Here's how the part is built. I have some questions about the finished solid (model axes, mm). A direction names the side the tool comes from. Round coordinates to 2 decimals unless told otherwise and drop trailing zeros. Order: outer loops, then holes, each group sorted by start corner. A loop starts at its lowest first (then second) coordinate and runs counter-clockwise, first axis right, second up. Notation, with made-up numbers: (-5.75, 13.25) - (22.25, 13.25) arc R10 cw to (22.25, 30.25) - close; hole circle Ø6 at (38, 62.5). An arc over 180 degrees is marked (long way). Answer as a JSON object with one key per item and string values.
```python
from build123d import *

# Parameters (mm, degrees)
F0_R         = 74.0650481318
F0_R_2       = 64.8450067866
F1_DEPTH     = 12.7
F2_DEPTH     = 7.62
F0_R_3       = 8.5707717009
F3_DEPTH     = 10.922
F4_R         = 5.08
F5_T4_DEPTH  = 123.6076762244
F5_T11_DEPTH = 122.6061545132
F5_T18_DEPTH = 115.6407516409


# Not quite as in the source:
# - a fillet or chamfer that OpenCascade refuses, or shapes differently, is made with other operations: its cross-section is extruded or revolved along the edge and cut away or added


with BuildPart() as f1:
    # F0 (on Top) → F1 (new body)
    with BuildSketch(Plane.XY):
        Circle(F0_R)
        Circle(F0_R_2, mode=Mode.SUBTRACT)
    extrude(amount=F1_DEPTH)

    # F0 (on Top) → F2 (join)
    with BuildSketch(Plane.XY):
        Circle(F0_R_2)
        Polygon((45.8412840962, -32.8662097454), (-43.6711683869, -32.8662097454), (0, 53.1617254019), align=None, mode=Mode.SUBTRACT)
    extrude(amount=F2_DEPTH)

    # F0 (on Top) → F3 (join)
    with BuildSketch(Plane.XY):
        Polygon((0, 53.1617254019), (-43.6711683869, -32.8662097454), (45.8412840962, -32.8662097454), align=None)
        Circle(F0_R_3, mode=Mode.SUBTRACT)
    extrude(amount=F3_DEPTH)

    # F4
    f4_edges = [f1.edges().sort_by_distance(p)[0] for p in [
        (-74.065048, 0, 12.7),
    ]]
    fillet(f4_edges, radius=F4_R)

    # F5: chamfer of 5.08 on 4 edges, made by hand


with BuildPart() as f5_tool2:
    # F5_s3 → F5_t4 (new body)
    with BuildSketch(Plane(origin=(29.9216472697, -56.1523871237, 0), x_dir=(0, 0, 1), z_dir=(-0.4702664859, 0.8825244655, 0))):
        Polygon((10.922, 19.9201777866), (5.842, 25.0001777866), (10.922, 25.0001777866), align=None)
    extrude(amount=F5_T4_DEPTH)

    split(bisect_by=Plane.XY.offset(7.62), keep=Keep.TOP)

    split(bisect_by=Plane(origin=(-21.4574493748, 10.8926464781, 0), x_dir=(0, 0, 1), z_dir=(0.8916858157, -0.4526548422, 0)), keep=Keep.TOP)

    split(bisect_by=Plane.XZ.offset(32.8662097454), keep=Keep.BOTTOM)


with BuildPart() as f1_1:
    add(f1.part)

    # F5_t1: cut F5_tool2
    add(f5_tool2.part, mode=Mode.SUBTRACT)


with BuildPart() as f5_tool9:
    # F5_s10 → F5_t11 (new body)
    with BuildSketch(Plane(origin=(27.3709999402, 53.9181957971, 0), x_dir=(0, 0, 1), z_dir=(-0.4526548422, -0.8916858157, 0))):
        Polygon((10.922, 18.9839124202), (5.842, 24.0639124202), (10.922, 24.0639124202), align=None)
    extrude(amount=F5_T11_DEPTH)

    split(bisect_by=Plane.XY.offset(7.62), keep=Keep.TOP)

    split(bisect_by=Plane(origin=(22.0632685396, 11.7567457534, 0), x_dir=(0, 0, 1), z_dir=(-0.8825244655, -0.4702664859, 0)), keep=Keep.TOP)

    split(bisect_by=Plane.XZ.offset(32.8662097454), keep=Keep.BOTTOM)


with BuildPart() as f1_2:
    add(f1_1.part)

    # F5_t8: cut F5_tool9
    add(f5_tool9.part, mode=Mode.SUBTRACT)


with BuildPart() as f5_tool16:
    # F5_s17 → F5_t18 (new body)
    with BuildSketch(Plane.YZ.offset(-56.7353179658)):
        Polygon((-27.7862097454, 10.922), (-32.8662097454, 5.842), (-32.8662097454, 10.922), align=None)
    extrude(amount=F5_T18_DEPTH)

    split(bisect_by=Plane.XY.offset(7.62), keep=Keep.TOP)

    split(bisect_by=Plane(origin=(22.0632685396, 11.7567457534, 0), x_dir=(0, 0, 1), z_dir=(-0.8825244655, -0.4702664859, 0)), keep=Keep.TOP)

    split(bisect_by=Plane(origin=(-21.4574493748, 10.8926464781, 0), x_dir=(0, 0, 1), z_dir=(0.8916858157, -0.4526548422, 0)), keep=Keep.TOP)


with BuildPart() as f1_3:
    add(f1_2.part)

    # F5_t15: cut F5_tool16
    add(f5_tool16.part, mode=Mode.SUBTRACT)

    # F5_s22 → F5_t23 (revolve, cut)
    with BuildSketch(Plane.XZ):
        Polygon((8.5707717009, 5.842), (13.6507717009, 10.922), (8.5707717009, 10.922), align=None)
    revolve(axis=Axis((0, 0, 10.922), (0, 0, 1)), mode=Mode.SUBTRACT)


solid = f1_3.part
```
1. Imagine slicing it at B-B (z = 3). List the corners of the cut face in (x, y) for me.
Responses:
{"outline": "circle Ø148.13 at (0, 0); hole circle Ø17.14 at (0, 0)"}
2. Imagine slicing it at A-A (y = 0). List the corners of the cut face in (x, z) for me (3 decimals), plus the area to 3 significant figures.
Responses:
{"outline": "(-74.065, 0) - (-8.571, 0) - (-8.571, 5.842) - (-13.651, 10.922) - (-21.29, 10.922) - (-24.993, 7.62) - (-64.845, 7.62) - (-64.845, 12.7) - (-68.985, 12.7) arc R5.08 ccw to (-74.065, 7.62) - close; (8.571, 0) - (74.065, 0) - (74.065, 7.62) arc R5.08 ccw to (68.985, 12.7) - (64.845, 12.7) - (64.845, 7.62) - (26.313, 7.62) - (22.572, 10.922) - (13.651, 10.922) - (8.571, 5.842) - close", "area": "1,160 mm2"}
3. For P1, Ø5, axis at y = -48, z = 7, coming from the -X side; P2, Ø1, axis at y = 43.5, z = 9.5, coming from the +X side; P3, Ø2, axis at x = 43.5, z = 5.5, coming from the +Y side; P4, Ø22.5, axis at x = 0, y = 0, coming from the -Z side, each with a flat end and sliding along its axis, tell me the tip position at first contact or that it passes through.
Responses:
{"P1": "x = -58.44", "P2": "x = 59.93", "P3": "y = 60.66", "P4": "z = 0"}
4. Thinking about a two-plate mould opening in X: for faces 3 (the face through (39.82, 62.45, 3.76)), 4 (the face through (-18.59, 8.92, 9.29)), 5 (the face through (51, -41, 12.7)), which applies, pulls with the +X half, pulls with the -X half, needs draft (parallel to the pull), parting line crosses it, or undercut?
Responses:
{"face 3": "parting line crosses it", "face 4": "undercut", "face 5": "needs draft"}
5. If I drill on L1, parallel to Y at x = 40, z = 8; L2, parallel to Y at x = -21.5, z = 8.5; L3, parallel to Y at x = 0, z = 3.3, over which ranges is the centre line in solid material (lowest first)? Write a range as [from, to].
Responses:
{"L1": "[-62.32, -51.04], [-30.71, -26.49], [51.04, 62.32]", "L2": "[-70.8, -61.18], [-30.21, 4.94], [61.18, 70.8]", "L3": "[-74.07, -8.57], [8.57, 74.07]"}
6. For faces 1 (the face through (15, 1, 0)), 2 (the face through (0, -16, 10.922)), which set-ups out of +Z, -Z, +X, -X, +Y, -Y let a thin tool reach every point of the face, with its end or its side?
Responses:
{"face 1": "-Z, +X, -X, +Y, -Y", "face 2": "+Z"}
